from build123d import *

# Parameters (mm, degrees)
F0_W     = 29
F0_H     = 79
F0_R     = 1.5
F0_R_2   = 1
F1_DEPTH = 9.5
F2_DEPTH = 10.5
F3_W     = 0.5
F3_H     = 13
F3_W_2   = 19
F3_H_2   = 0.5
F4_DEPTH = 77
F5_DEPTH = 79
F6_DEPTH = 8
F7_DEPTH = 5
F8_SIZE2 = 0.49999
F8_SIZE  = 0.49999


# Not quite as in the source:
# - a fillet or chamfer is up to 0.001 mm smaller than in the source, because OpenCascade refuses the exact size


with BuildPart() as f1:
    # F0 (on Top) → F1 (new body, symmetric)
    with BuildSketch(Plane.XY):
        with Locations((0, 39.5)):
            Rectangle(F0_W, F0_H)
        with Locations((-12, 3)):
            Circle(F0_R, mode=Mode.SUBTRACT)
        with Locations((-12, 16)):
            Circle(F0_R_2, mode=Mode.SUBTRACT)
        with Locations((12, 3)):
            Circle(F0_R, mode=Mode.SUBTRACT)
        with Locations((12, 16)):
            Circle(F0_R_2, mode=Mode.SUBTRACT)
    extrude(amount=F1_DEPTH, both=True)

    # F0 (on Top) → F2 (join, symmetric)
    with BuildSketch(Plane.XY):
        with Locations((-12, 3)):
            Circle(F0_R)
        with Locations((12, 3)):
            Circle(F0_R)
    extrude(amount=F2_DEPTH, both=True)

    # F3 (on Front) → F4 (cut)
    with BuildSketch(Plane.XZ):
        Polygon((9.5, 9), (-9.5, 9), (-14, 9), (-14, 6.5), (-14, -6.5), (-14, -9), (-9.5, -9), (9.5, -9), (14, -9), (14, -6.5), (14, 6.5), (14, 9), align=None)
        with Locations((-14.25, 0)):
            Rectangle(F3_W, F3_H)
        with Locations((0, 9.25)):
            Rectangle(F3_W_2, F3_H_2)
        with Locations((14.25, 0)):
            Rectangle(F3_W, F3_H)
        with Locations((0, -9.25)):
            Rectangle(F3_W_2, F3_H_2)
    extrude(amount=-F4_DEPTH, mode=Mode.SUBTRACT)

    # F3 (on Front) → F5 (cut)
    with BuildSketch(Plane.XZ):
        Polygon((9.5, 9), (-9.5, 9), (-14, 9), (-14, 6.5), (-14, -6.5), (-14, -9), (-9.5, -9), (9.5, -9), (14, -9), (14, -6.5), (14, 6.5), (14, 9), align=None)
        with Locations((-14.25, 0)):
            Rectangle(F3_W, F3_H)
        with Locations((14.25, 0)):
            Rectangle(F3_W, F3_H)
    extrude(amount=-F5_DEPTH, mode=Mode.SUBTRACT)

    # F3 (on Front) → F6 (join)
    with BuildSketch(Plane.XZ):
        with Locations((-14.25, 0)):
            Rectangle(F3_W, F3_H)
        with Locations((14.25, 0)):
            Rectangle(F3_W, F3_H)
    extrude(amount=-F6_DEPTH)

    # F3 (on Front) → F7 (cut)
    with BuildSketch(Plane.XZ):
        with Locations((-14.25, 0)):
            Rectangle(F3_W, F3_H)
        with Locations((14.25, 0)):
            Rectangle(F3_W, F3_H)
    extrude(amount=-F7_DEPTH, mode=Mode.SUBTRACT)

    # F8 (size 0.5 and 0.5 in the source; OpenCascade refuses exactly that, so slightly less here)
    f8_edges = [f1.edges().sort_by_distance(p)[0] for p in [
        (-9.5, 38.5, -9),
        (9.5, 38.5, -9),
        (14, 43.5, -6.5),
        (-14, 43.5, -6.5),
        (14, 43.5, 6.5),
        (9.5, 38.5, 9),
        (-14, 43.5, 6.5),
        (-9.5, 38.5, 9),
        (14.5, 0, -8),
        (14.5, 0, 8),
        (-14.5, 0, -8),
        (-14.5, 0, 8),
        (-14, 5, 0),
        (14, 5, 0),
        (-14, 8, 0),
        (14, 8, 0),
        (0, 77, -9),
        (0, 77, 9),
    ]]
    chamfer(f8_edges, length=F8_SIZE, length2=F8_SIZE2)


solid = f1.part
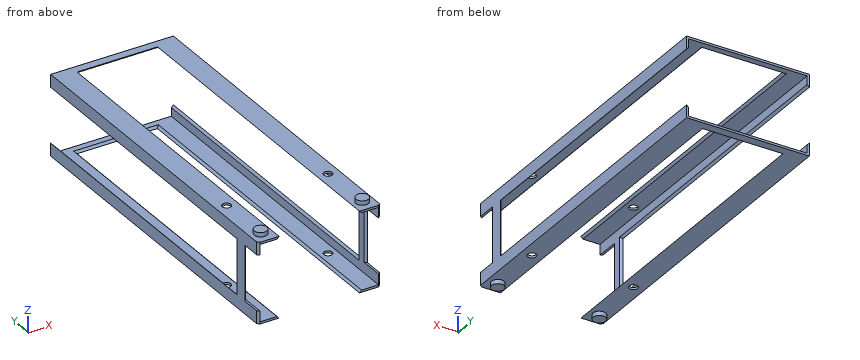
Part model, mm, in its own coordinate system. Round coordinates to 2 decimals unless told otherwise and drop trailing zeros. Write each loop counter-clockwise with the first axis right and the second up, starting at its lowest first coordinate (ties: lowest second). Pieces come first, ordered by that corner, then holes. Notation, with made-up numbers: M -24.75,70.25 L -10.75,70.25 A19 cw -10.75,100.25 Z; hole C 46,83.25 d2. An arc over 180 degrees is marked long. Return JSON: item names as keys, results as strings. Group by question number.
(1) Saw through at B-B on y = 22.5. Count the separate pieces of the cut face and the enclosed holes in it, then the cut area to 3 significant figures.
(2) Pin check, flat tips, straight feed: pin 1 Ø6 at (x, y) = (-7.5, 54) entering from +Z; pin 2 Ø3 at (x, y) = (-12, 16) entering from -Z; pin 3 Ø8.5 at (x, y) = (5, 30.5) entering from +Z. Stop position of each tip, or through.
(3) Drill centre lines: probe 1 along X at (y, z) = (16.5, 8.75); probe 2 along Z at (x, y) = (-11.25, 21); probe 3 along Y at (x, z) = (-12, 9.25). Where is each one in solid material? Low to high.
(4) Saw through at D-D on x = 12. Write the cut outline in (y, z).
Returned:
{
 "1": {"separate pieces": "4", "enclosed holes": "0", "area": "14.0 mm²"},
 "2": {"pin 1": "z = 9.5", "pin 2": "z = -9.5", "pin 3": "through"},
 "3": {"probe 1": "-14.5 to -14, 14 to 14.5", "probe 2": "-9.5 to -9, 9 to 9.5", "probe 3": "0 to 15, 17 to 79"},
 "4": {"outline": "M 0,-9.5 L 1.5,-9.5 L 1.5,-10.5 L 4.5,-10.5 L 4.5,-9.5 L 15,-9.5 L 15,-9 L 0,-9 Z; M 0,9 L 15,9 L 15,9.5 L 4.5,9.5 L 4.5,10.5 L 1.5,10.5 L 1.5,9.5 L 0,9.5 Z; M 17,-9.5 L 79,-9.5 L 79,-9 L 17,-9 Z; M 17,9 L 79,9 L 79,9.5 L 17,9.5 Z"}
}
